The listing builds one solid part. Answer for the finished solid, in the listing's coordinates (mm). A direction names the side the tool comes from. Round coordinates to 2 decimals unless told otherwise and drop trailing zeros. Order: outer loops, then holes, each group sorted by start corner. A loop starts at its lowest first (then second) coordinate and runs counter-clockwise, first axis right, second up. Notation, with made-up numbers: (59.25, 14.25) - (114.25, 14.25) arc R14 cw to (114.25, 21.25) - close; hole circle Ø7 at (58, 69). An arc over 180 degrees is marked (long way). Write item = value, one per line.
from build123d import *

# Parameters (mm, degrees)
F0_R      = 9.525
F1_DEPTH  = 8.6995
F2_R      = 11.1125
F3_DEPTH  = 7.112
F4_T      = -3.175
F5_R      = 3.175
F6_W      = 16.66875
F6_H      = 16.66875
F7_DEPTH  = 5.5245
F8_R      = 8.334375
F9_R      = 6.746875
F10_DEPTH = 7.9375
F11_R     = 2.15265
F12_DEPTH = 8.6995


with BuildPart() as f1:
    # F0 (on Top) → F1 (new body)
    with BuildSketch(Plane.XY):
        with BuildLine():
            Line((-14.2875, 369.1638474552), (-14.2875, 0))
            ThreePointArc((-14.2875, 0), (-13.1999288208, -5.4675895399), (-10.1027881362, -10.1027881362))
            Line((-10.1027881362, -10.1027881362), (23.8125, -44.0180762724))
            Line((23.8125, -44.0180762724), (74.6125, -44.0180762724))
            Line((74.6125, -44.0180762724), (74.6125, 413.1819237276))
            Line((74.6125, 413.1819237276), (23.8125, 413.1819237276))
            Line((23.8125, 413.1819237276), (-10.1027881362, 379.2666355914))
            ThreePointArc((-10.1027881362, 379.2666355914), (-13.1999288208, 374.6314369951), (-14.2875, 369.1638474552))
        make_face()
        Circle(F0_R, mode=Mode.SUBTRACT)
        with Locations((0, 369.1638474552)):
            Circle(F0_R, mode=Mode.SUBTRACT)
    extrude(amount=F1_DEPTH)

    # F2 (on face) → F3 (cut)
    with BuildSketch(Plane.XY.offset(8.6995)):
        with Locations((0, 369.1638474552)):
            Circle(F2_R)
        Circle(F2_R)
    extrude(amount=-F3_DEPTH, mode=Mode.SUBTRACT)

    # F4
    f4_openings = [f1.faces().sort_by_distance(p)[0] for p in [
        (31.981731, 184.581924, 8.6995),
    ]]
    offset(amount=F4_T, openings=f4_openings)

    # F5
    f5_edges = [f1.edges().sort_by_distance(p)[0] for p in [
        (-1.507724, 383.371572, 5.93725),
        (-11.1125, 360.183591, 5.93725),
        (-11.1125, 8.980256, 5.93725),
        (-1.507724, -14.207724, 5.93725),
    ]]
    fillet(f5_edges, radius=F5_R)

    # F6 (on face) → F7 (join, through all)
    with BuildSketch(Plane.XY.offset(3.175)):
        with Locations((66.278125, 404.8475487276)):
            Rectangle(F6_W, F6_H)
        with Locations((66.278125, -35.6837012724)):
            Rectangle(F6_W, F6_H)
    extrude(amount=F7_DEPTH)

    # F8
    f8_edges = [f1.edges().sort_by_distance(p)[0] for p in [
        (74.6125, 413.181924, 4.34975),
        (74.6125, -44.018076, 4.34975),
        (57.94375, -27.349326, 5.93725),
        (57.94375, 396.513174, 5.93725),
    ]]
    fillet(f8_edges, radius=F8_R)

    # F9 (on face) → F10 (cut)
    with BuildSketch(Plane(origin=(0, 0, 0), x_dir=(1, 0, 0), z_dir=(0, 0, -1))):
        with Locations((66.278125, 35.6837012724)):
            Circle(F9_R)
        with Locations((66.278125, -404.8475487276)):
            Circle(F9_R)
    extrude(amount=-F10_DEPTH, mode=Mode.SUBTRACT)

    # F11 (on face) → F12 (cut, through all)
    with BuildSketch(Plane(origin=(0, 0, 0), x_dir=(1, 0, 0), z_dir=(0, 0, -1))):
        with Locations((66.278125, 35.6837012724)):
            Circle(F11_R)
        with Locations((66.278125, -404.8475487276)):
            Circle(F11_R)
    extrude(amount=-F12_DEPTH, mode=Mode.SUBTRACT)


solid = f1.part
Q1. Flat-ended cylindrical pins translate along their axes: P1, Ø12, axis at x = 10.5, y = 224.5, coming from the +Z side (3 decimals); P2, Ø4, axis at y = -38, z = 5.5, coming from the -X side; P3, Ø4, axis at y = 408, z = 7, coming from the -X side. Find the tip coordinate at first contact, or state that the pin passes through.
Model answer:
P1 = 3.175
P2 = 15.79
P3 = 16.63
Q2. Section A-A on x = 52.5 is taken. Determine the outline of the cut face in (y, z) (1 decimal), then the cut area to 3 significant figures.
Model answer:
outline = (-44, 0) - (413.2, 0) - (413.2, 8.7) - (410, 8.7) - (410, 3.2) - (-40.8, 3.2) - (-40.8, 8.7) - (-44, 8.7) - close
area = 1,490 mm^2
Q3. Determine the mould class of faces 1 (the face through (-13.23, -5.39, 4.29)), 2 (the face through (14.29, 399.17, 5.9)), 3 (the face through (7.09, 396.46, 4.29)) for opening direction Y: released by +Y, released by -Y, zero draft, split by the parting line, or undercut.
Model answer:
face_1 = released by -Y
face_2 = undercut
face_3 = released by +Y
Q4. Section C-C on z = 5.5 is taken. Count the separate pieces of the cut face and the enclosed holes in it, then the cut area to 3 significant figures.
Model answer:
separate_pieces = 1
enclosed_holes = 5
area = 3,700 mm^2
Q5. For faces 4 (the face through (66, 408, 7.938)), 5 (the face through (60.45, -29.726, 5.976)), 6 (the face through (-1.24, 378.608, 0.783)), determine the directions among +Z, -Z, +X, -X, +Y, -Y from which every point of the face is accessible in a straight line to the end or side of a thin tool.
Model answer:
face_4 = -Z
face_5 = +Z
face_6 = +Z, -Z
Q6. Section B-B on y = 342 is taken. Determine the outline of the cut face in (x, z) (1 decimal), then the cut area to 3 significant figures.
Model answer:
outline = (-14.3, 0) - (74.6, 0) - (74.6, 8.7) - (71.4, 8.7) - (71.4, 3.2) - (-11.1, 3.2) - (-11.1, 8.7) - (-14.3, 8.7) - close
area = 317 mm^2
Q7. Find the intervals of material crossed by line 1 (X direction, y = 52, z = 5.75); line 2 (Y direction, x = 33, z = 7); line 3 (X direction, y = 9, z = 7), in increasing order. Write a range as from..to.
Model answer:
line_1 = -14.29..-11.11, 71.44..74.61
line_2 = -44.02..-40.84, 410.01..413.18
line_3 = -14.29..-6.52, 6.52..11.1, 71.44..74.61
